For this review, take the finished solid that the model builds, in its own axes (mm). A direction names the side the tool comes from. Give positions to 0.01 mm unless a question says otherwise; leave off trailing zeros. Loops run counter-clockwise (first coordinate to the right, second up) from the corner with the lowest first, then second, coordinate; pieces in that order, holes last. Notation, with made-up numbers: (47, 57.25) -> (96, 57.25) arc R26 cw to (96, 71.25) -> close; hole circle Ø6 at (-19, 83.5). An arc over 180 degrees is marked (long way). Answer as CSV lines item,"result". Start each with the question number.
Item 1: Machinability: for faces 1 (the face through (-9, 2, 5)), 2 (the face through (0, 1.5, 4)), 3 (the face through (9, 2, 5)), 4 (the face through (-2, -6, 13)), which of the approach directions +Z, -Z, +X, -X, +Y, -Y give a long, thin tool a straight path to every point of the face, cutting with its end or side? Answer none if there is none.
Item 2: Add section C-C on y = -3. State the section outline as (x, z) points, plus the area to 3 significant figures.
Item 3: Clearance check with flat-ended pins moving along their axes: P1, Ø4, axis at x = -7.5, z = 5, coming from the +Y side; P2, Ø1.5, axis at x = -7.5, y = -6.5, coming from the -Z side; P3, Ø4, axis at y = -7, z = 13.5, coming from the -X side; P4, Ø2.5, axis at x = 1.5, z = 6, coming from the -Y side. State where each tip first meets the part, or that it passes through.
Item 4: Add section B-B on x = 0. State the section outline as (y, z) points, plus the area to 3 significant figures.
Item 5: Add section A-A on z = 5.75. State the section outline as (x, y) points, plus the area to 3 significant figures.
Item 6: For L1, parallel to Y at x = 0, z = 9; L2, parallel to Y at x = 1.5, z = 7.5; L3, parallel to X at y = -3.75, z = 4, list the stretches that pass through material, from the lowest coordinate up. Write a range as from..to.
Item 7: Add section D-D on z = 13.25. State the section outline as (x, y) points.
```python
from build123d import *

# Parameters (mm, degrees)
F1_DEPTH = 10
F2_DEPTH = 15
F3_W     = 8
F3_H     = 3
F4_DEPTH = 8
F5_R     = 2
F6_DEPTH = 25
F8_DEPTH = 5


with BuildPart() as f1:
    # F0 (on Top) → F1 (new body)
    with BuildSketch(Plane.XY):
        with BuildLine():
            Line((-8.7749643874, 2), (-9.7979589711, 2))
            ThreePointArc((-9.7979589711, 2), (-10, 0), (-9.7979589711, -2))
            Line((-9.7979589711, -2), (-8.7749643874, -2))
            ThreePointArc((-8.7749643874, -2), (-9, 0), (-8.7749643874, 2))
        make_face()
        with BuildLine():
            ThreePointArc((9.7979589711, -2), (9.9493615301, -1.0050896201), (10, 0))
            ThreePointArc((10, 0), (9.9493615301, 1.0050896201), (9.7979589711, 2))
            Line((9.7979589711, 2), (8.7749643874, 2))
            ThreePointArc((8.7749643874, 2), (8.9435641521, 1.0063102189), (9, 0))
            ThreePointArc((9, 0), (8.9435641521, -1.0063102189), (8.7749643874, -2))
            Line((8.7749643874, -2), (9.7979589711, -2))
        make_face()
        with BuildLine():
            ThreePointArc((9, 0), (8.9435641521, 1.0063102189), (8.7749643874, 2))
            Line((8.7749643874, 2), (-8.7749643874, 2))
            ThreePointArc((-8.7749643874, 2), (-9, 0), (-8.7749643874, -2))
            Line((-8.7749643874, -2), (8.7749643874, -2))
            ThreePointArc((8.7749643874, -2), (8.9435641521, -1.0063102189), (9, 0))
        make_face()
        with BuildLine():
            Line((-8.7749643874, 2), (8.7749643874, 2))
            ThreePointArc((8.7749643874, 2), (0, 9), (-8.7749643874, 2))
        make_face()
        with BuildLine():
            ThreePointArc((-8.7749643874, -2), (0, -9), (8.7749643874, -2))
            Line((8.7749643874, -2), (-8.7749643874, -2))
        make_face()
    extrude(amount=F1_DEPTH)

    # F0 (on Top) → F2 (join)
    with BuildSketch(Plane.XY):
        with BuildLine():
            ThreePointArc((9, 0), (8.9435641521, 1.0063102189), (8.7749643874, 2))
            Line((8.7749643874, 2), (-8.7749643874, 2))
            ThreePointArc((-8.7749643874, 2), (-9, 0), (-8.7749643874, -2))
            Line((-8.7749643874, -2), (8.7749643874, -2))
            ThreePointArc((8.7749643874, -2), (8.9435641521, -1.0063102189), (9, 0))
        make_face()
        with BuildLine():
            Line((-8.7749643874, 2), (8.7749643874, 2))
            ThreePointArc((8.7749643874, 2), (0, 9), (-8.7749643874, 2))
        make_face()
        with BuildLine():
            ThreePointArc((-8.7749643874, -2), (0, -9), (8.7749643874, -2))
            Line((8.7749643874, -2), (-8.7749643874, -2))
        make_face()
    extrude(amount=F2_DEPTH)

    # F3 (on face) → F4 (cut)
    with BuildSketch(Plane.XY):
        Rectangle(F3_W, F3_H)
    extrude(amount=F4_DEPTH, mode=Mode.SUBTRACT)

    # F5 (on face) → F6 (cut)
    with BuildSketch(Plane.XY.offset(15)):
        with Locations((0, -4)):
            Circle(F5_R)
    extrude(amount=-F6_DEPTH, mode=Mode.SUBTRACT)

    # F7 (on face) → F8 (cut)
    with BuildSketch(Plane.XY.offset(15)):
        with BuildLine():
            ThreePointArc((1.9984808879, -4.0779367749), (-0.0179678096, -5.9999192878), (-1.9995585875, -4.0420173194))
            Line((-1.9995585875, -4.0420173194), (-1.9995585875, -8.775064983))
            ThreePointArc((-1.9995585875, -8.775064983), (-0.0005526547, -8.999999983), (1.9984808879, -8.7753104869))
            Line((1.9984808879, -8.7753104869), (1.9984808879, -4.0779367749))
        make_face()
    extrude(amount=-F8_DEPTH, mode=Mode.SUBTRACT)


solid = f1.part
```
Computed values:
1,face 1,"+Z, -Z, -X, +Y"
1,face 2,"-Z"
1,face 3,"+Z, -Z, +X, +Y"
1,face 4,"+Z, -Y"
2,outline,"(-8.49, 0) -> (-1.73, 0) -> (-1.73, 15) -> (-8.49, 15) -> close; (1.73, 0) -> (8.49, 0) -> (8.49, 15) -> (1.73, 15) -> close"
2,area,"203 mm²"
3,P1,"y = 7.12"
3,P2,"through"
3,P3,"x = -7.48"
3,P4,"y = -9"
4,outline,"(-9, 0) -> (-6, 0) -> (-6, 10) -> (-9, 10) -> close; (-2, 0) -> (-1.5, 0) -> (-1.5, 8) -> (1.5, 8) -> (1.5, 0) -> (9, 0) -> (9, 15) -> (-2, 15) -> close"
4,area,"171 mm²"
5,outline,"(-9.8, -2) -> (-8.77, -2) arc R9 ccw to (8.77, -2) -> (9.8, -2) arc R10 ccw to (9.8, 2) -> (8.77, 2) arc R9 ccw to (-8.77, 2) -> (-9.8, 2) arc R10 ccw to start; hole (-4, -1.5) -> (4, -1.5) -> (4, 1.5) -> (-4, 1.5) -> close; hole circle Ø4 at (0, -4)"
5,area,"226 mm²"
6,L1,"-9..-6, -2..9"
6,L2,"-8.87..-5.32, -2.68..-1.5, 1.5..8.87"
6,L3,"-8.18..-1.98, 1.98..8.18"
7,outline,"(-2, -8.78) -> (-2, -4.04) arc R2 cw (long way) to (2, -4.08) -> (2, -8.78) arc R9 ccw (long way) to start"
